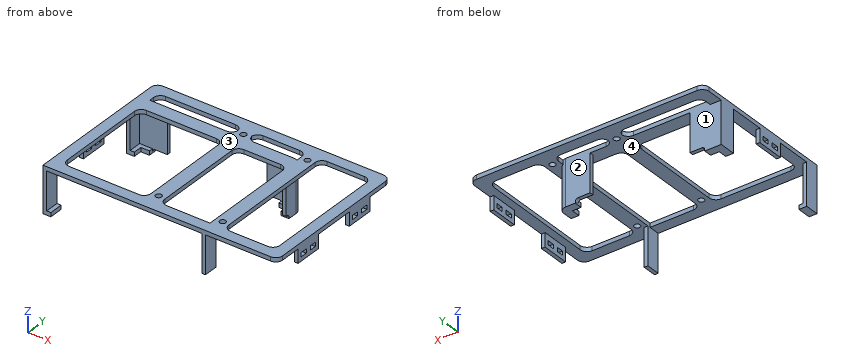
```python
from build123d import *

# Parameters (mm, degrees)
SKETCH1_W               = 170.3
SKETCH1_H               = 110
SKETCH1_W_2             = 60.75
SKETCH1_H_2             = 75.3
SKETCH1_H_3             = 8.7
SKETCH1_W_3             = 37
SKETCH1_H_4             = 94
SKETCH1_W_4             = 36.55
BOSS_EXTRUDE1_DEPTH     = 3
F_6_CLEARANCE_HOLE1_D   = 4.3053
SKETCH6_W               = 2.7
SKETCH6_H               = 10
BOSS_EXTRUDE2_DEPTH     = 27.6
SKETCH7_W               = 5.7
SKETCH7_H               = 10
BOSS_EXTRUDE3_DEPTH     = 3
FILLET3_R               = 5
FILLET4_R               = 2
FILLET5_R               = 5
SKETCH8_W               = 2.7
SKETCH8_H               = 20
BOSS_EXTRUDE4_DEPTH     = 10
CUT_EXTRUDE1_DEPTH      = 206.032802254
CUT_EXTRUDE1_DEPTH_BACK = 3
SKETCH9_W               = 3
SKETCH9_H               = 5
SKETCH11_W              = 2.7
SKETCH11_H              = 20
BOSS_EXTRUDE5_DEPTH     = 10
SKETCH12_W              = 3
SKETCH12_H              = 5
CUT_EXTRUDE2_DEPTH      = 3


with BuildPart() as part:
    # Sketch1 → Boss-Extrude1 (new body)
    with BuildSketch(Plane.XY):
        with Locations((85.15, 55)):
            Rectangle(SKETCH1_W, SKETCH1_H)
        with Locations((38.375, 45.65)):
            Rectangle(SKETCH1_W_2, SKETCH1_H_2, mode=Mode.SUBTRACT)
        with Locations((38.375, 97.65)):
            Rectangle(SKETCH1_W_2, SKETCH1_H_3, mode=Mode.SUBTRACT)
        with Locations((143.8, 55)):
            Rectangle(SKETCH1_W_3, SKETCH1_H_4, mode=Mode.SUBTRACT)
        with Locations((97.025, 45.65)):
            Rectangle(SKETCH1_W_4, SKETCH1_H_2, mode=Mode.SUBTRACT)
        with Locations((97.025, 97.65)):
            Rectangle(SKETCH1_W_4, SKETCH1_H_3, mode=Mode.SUBTRACT)
    extrude(amount=BOSS_EXTRUDE1_DEPTH)

    # #6 Clearance Hole1 (through all)
    with Locations(Plane(origin=(0, 0, 0), x_dir=(-1, 0, 0), z_dir=(0, 0, -1))):
        with Locations((-120.3, 13.725), (-120.3, 96.275), (-73.75, 13.725), (-73.75, 96.275)):
            Hole(F_6_CLEARANCE_HOLE1_D / 2)

    # Sketch6 → Boss-Extrude2 (add)
    with BuildSketch(Plane(origin=(0, 0, 0), x_dir=(-1, 0, 0), z_dir=(0, 0, -1))):
        with Locations((-1.35, 5)):
            Rectangle(SKETCH6_W, SKETCH6_H)
        with Locations((-116.65, 5)):
            Rectangle(SKETCH6_W, SKETCH6_H)
        Polygon((0, 81.3), (0, 93.3), (-22.7, 93.3), (-22.7, 90.6), (-2.7, 90.6), (-2.7, 81.3), align=None)
        Polygon((-95.3, 93.3), (-118, 93.3), (-118, 78.6), (-115.3, 78.6), (-115.3, 90.6), (-95.3, 90.6), align=None)
    extrude(amount=BOSS_EXTRUDE2_DEPTH)

    # Sketch7 → Boss-Extrude3 (add)
    with BuildSketch(Plane(origin=(0, 0, -27.6), x_dir=(-1, 0, 0), z_dir=(0, 0, -1))):
        Polygon((0, 93.3), (0, 81.3), (-5.7, 81.3), (-5.7, 87.6), (-12, 87.6), (-12, 93.3), align=None)
        with Locations((-2.85, 5)):
            Rectangle(SKETCH7_W, SKETCH7_H)
        Polygon((-118, 93.3), (-118, 81.3), (-112.3, 81.3), (-112.3, 87.6), (-106, 87.6), (-106, 93.3), align=None)
    extrude(amount=BOSS_EXTRUDE3_DEPTH)

    # Fillet3
    fillet3_edges = [part.edges().sort_by_distance(p)[0] for p in [
        (118, 93.3, -15.3),
    ]]
    fillet(fillet3_edges, radius=FILLET3_R)

    # Fillet4
    fillet4_edges = [part.edges().sort_by_distance(p)[0] for p in [
        (12, 91.95, -27.6),
        (106, 91.95, -27.6),
        (116.65, 81.3, -27.6),
    ]]
    fillet(fillet4_edges, radius=FILLET4_R)

    # Fillet5
    # the kernel refuses this fillet: 5 mm, written as the material it adds along each edge
    with BuildSketch(Plane(origin=(8, 83.3, 0), x_dir=(0, -1, 0), z_dir=(0, 0, 1)), Plane(origin=(68.75, 83.3, 0), x_dir=(-1, 0, 0), z_dir=(0, 0, 1)), Plane(origin=(125.3, 102, 0), x_dir=(0, -1, 0), z_dir=(0, 0, 1)), Plane(origin=(125.3, 8, 0), x_dir=(1, 0, 0), z_dir=(0, 0, 1)), Plane(origin=(68.75, 93.3, 0), x_dir=(0, 1, 0), z_dir=(0, 0, 1)), Plane(origin=(68.75, 102, 0), x_dir=(-1, 0, 0), z_dir=(0, 0, 1)), Plane(origin=(78.75, 8, 0), x_dir=(1, 0, 0), z_dir=(0, 0, 1)), Plane(origin=(78.75, 102, 0), x_dir=(0, -1, 0), z_dir=(0, 0, 1)), Plane(origin=(78.75, 93.3, 0), x_dir=(1, 0, 0), z_dir=(0, 0, 1))) as fillet5_piece_1:
        with BuildLine():
            CenterArc((FILLET5_R, FILLET5_R), FILLET5_R, 180, 90)
            Line((0, FILLET5_R), (0, 0))
            Line((0, 0), (FILLET5_R, 0))
        make_face()
    extrude(amount=3)
    with BuildSketch(Plane(origin=(8, 8, 0), x_dir=(0, 1, 0), z_dir=(0, 0, 1)), Plane(origin=(68.75, 8, 0), x_dir=(-1, 0, 0), z_dir=(0, 0, 1)), Plane(origin=(162.3, 102, 0), x_dir=(0, -1, 0), z_dir=(0, 0, 1)), Plane(origin=(162.3, 8, 0), x_dir=(-1, 0, 0), z_dir=(0, 0, 1)), Plane(origin=(8, 102, 0), x_dir=(1, 0, 0), z_dir=(0, 0, 1)), Plane(origin=(115.3, 83.3, 0), x_dir=(0, -1, 0), z_dir=(0, 0, 1)), Plane(origin=(78.75, 83.3, 0), x_dir=(1, 0, 0), z_dir=(0, 0, 1)), Plane(origin=(115.3, 102, 0), x_dir=(0, -1, 0), z_dir=(0, 0, 1))) as fillet5_piece_2:
        with BuildLine():
            CenterArc((FILLET5_R, -FILLET5_R), FILLET5_R, 90, 90)
            Line((0, -FILLET5_R), (0, 0))
            Line((0, 0), (FILLET5_R, 0))
        make_face()
    extrude(amount=3)
    # the kernel refuses this fillet: 5 mm, written as the material it takes off along each edge
    with BuildSketch(Plane(origin=(0, 110, -12.5), x_dir=(0, -1, 0), z_dir=(0, 0, 1)), Plane(origin=(170.3, 110, -12.5), x_dir=(-1, 0, 0), z_dir=(0, 0, 1)), Plane(origin=(170.3, 0, -12.5), x_dir=(0, 1, 0), z_dir=(0, 0, 1))) as fillet5_2_piece_1:
        with BuildLine():
            CenterArc((FILLET5_R, FILLET5_R), FILLET5_R, 180, 90)
            Line((0, FILLET5_R), (0, 0))
            Line((0, 0), (FILLET5_R, 0))
        make_face()
    extrude(amount=28, mode=Mode.SUBTRACT)

    # Sketch8 → Boss-Extrude4 (add)
    with BuildSketch(Plane(origin=(0, 0, 0), x_dir=(-1, 0, 0), z_dir=(0, 0, -1))):
        with Locations((-1.35, 45.65)):
            Rectangle(SKETCH8_W, SKETCH8_H)
    extrude(amount=BOSS_EXTRUDE4_DEPTH)

    # Sketch9 → Cut-Extrude1 (cut, two sides: drawn at the far end of the back side and taken through both)
    with BuildSketch(Plane.ZY.offset(-CUT_EXTRUDE1_DEPTH_BACK)):
        with Locations((-5.5, 41.15)):
            Rectangle(SKETCH9_W, SKETCH9_H)
        with Locations((-5.5, 50.15)):
            Rectangle(SKETCH9_W, SKETCH9_H)
    extrude(amount=CUT_EXTRUDE1_DEPTH + CUT_EXTRUDE1_DEPTH_BACK, mode=Mode.SUBTRACT)

    # Sketch11 → Boss-Extrude5 (add)
    with BuildSketch(Plane(origin=(0, 0, 0), x_dir=(-1, 0, 0), z_dir=(0, 0, -1))):
        with Locations((-168.95, 30)):
            Rectangle(SKETCH11_W, SKETCH11_H)
        with Locations((-168.95, 80)):
            Rectangle(SKETCH11_W, SKETCH11_H)
    extrude(amount=BOSS_EXTRUDE5_DEPTH)

    # Sketch12 → Cut-Extrude2 (cut)
    with BuildSketch(Plane(origin=(170.3, 0, 0), x_dir=(0, 0, -1), z_dir=(1, 0, 0))):
        with Locations((5.5, 34.5)):
            Rectangle(SKETCH12_W, SKETCH12_H)
        with Locations((5.5, 25.5)):
            Rectangle(SKETCH12_W, SKETCH12_H)
        with Locations((5.5, 84.5)):
            Rectangle(SKETCH12_W, SKETCH12_H)
        with Locations((5.5, 75.5)):
            Rectangle(SKETCH12_W, SKETCH12_H)
    extrude(amount=-CUT_EXTRUDE2_DEPTH, mode=Mode.SUBTRACT)


solid = part.part
```
Input: part model. Units: mm. Frame: model coordinates. Face numbers are marked on the shaded views. A direction names the side the tool comes from. Give positions to 0.01 mm unless a question says otherwise; leave off trailing zeros. Loops run counter-clockwise (first coordinate to the right, second up) from the corner with the lowest first, then second, coordinate; pieces in that order, holes last. Notation, with made-up numbers: M -29,65 L 23,65 A14 cw 23,82 Z; hole C 12,79.5 d6. An arc over 180 degrees is marked long. Answer as CSV lines item,"result". Start each with the question number.
1. Line query: L1, parallel to Y at x = 120, z = 1; L2, parallel to X at y = 88, z = -13; L3, parallel to X at y = 68.5, z = 1.5. Output: solid intervals per line, ascending.
2. Pull-direction query (X, two-part tool) for the marked faces 3 and 4; classes: released by +X, released by -X, zero draft, split by the parting line, or undercut.
3. Section A-A on x = 101. Return loops of the section in (y, z), plus the area to 3 significant figures.
4. Reachability of the marked faces 1 and 2 from +Z, -Z, +X, -X, +Y, -Y: full face, straight path, thin tool, end or side. Return the list, or none.
5. Section D-D on x = 31.5. Return loops of the section in (y, z), plus the area to 3 significant figures.
6. Section B-B on x = 149. Return loops of the section in (y, z), plus the area to 3 significant figures.
7. Pin query (flat end, axial travel): P1, Ø1.3, axis at x = 169.5, z = -7, coming from the +Y side; P2, Ø8, axis at y = 6.5, z = -8, coming from the +X side; P3, Ø2, axis at x = 169, y = 28, coming from the -Z side; P4, Ø12, axis at y = 42, z = -19, coming from the -X side. Return the tip coordinate at first contact, or that it passes through.
8. Section C-C on z = -23.5. Return loops of the section in (x, y), plus the area to 3 significant figures.
Computed values:
1,L1,"y = 0 to 11.59, 15.86 to 94.14, 98.41 to 110"
1,L2,"x = 0 to 2.7, 115.3 to 118"
1,L3,"x = 0 to 8, 68.75 to 78.75, 115.3 to 125.3, 162.3 to 170.3"
2,face 3,"zero draft"
2,face 4,"undercut"
3,outline,"M 0,0 L 8,0 L 8,3 L 0,3 Z; M 83.3,0 L 90.6,0 L 90.6,-27.6 L 93.3,-27.6 L 93.3,3 L 83.3,3 Z; M 102,0 L 110,0 L 110,3 L 102,3 Z"
3,area,"153 mm²"
4,face 1,"-Z"
4,face 2,"+Z, -Z"
5,outline,"M 0,0 L 8,0 L 8,3 L 0,3 Z; M 83.3,0 L 93.3,0 L 93.3,3 L 83.3,3 Z; M 102,0 L 110,0 L 110,3 L 102,3 Z"
5,area,"78.0 mm²"
6,outline,"M 0,0 L 8,0 L 8,3 L 0,3 Z; M 102,0 L 110,0 L 110,3 L 102,3 Z"
6,area,"48.0 mm²"
7,P1,"stops at y = 90"
7,P2,"stops at x = 118"
7,P3,"stops at z = -10"
7,P4,"passes through"
8,outline,"M 0,0 L 2.7,0 L 2.7,10 L 0,10 Z; M 0,81.3 L 2.7,81.3 L 2.7,90.6 L 22.7,90.6 L 22.7,93.3 L 0,93.3 Z; M 95.3,90.6 L 115.3,90.6 L 115.3,78.6 L 118,78.6 L 118,88.3 A5 ccw 113,93.3 L 95.3,93.3 Z; M 115.3,0 L 118,0 L 118,10 L 115.3,10 Z"
8,area,"229 mm²"
